The model under review builds one solid part; all positions refer to its coordinate system, in mm. Coordinates: 2 decimals unless noted, no trailing zeros. Loops run counter-clockwise (first coordinate to the right, second up) from the corner with the lowest first, then second, coordinate; pieces in that order, holes last. Notation, with made-up numbers: M 29,23 L 54,23 A32 cw 54,52 Z; hole C 27,-23 d9. An arc over 180 degrees is marked long. Use one line per item in the form item = value.
```python
from build123d import *

# Parameters (mm, degrees)
SKETCH1_R                                       = 50
BOSS_EXTRUDE1_DEPTH                             = 5
SKETCH3_R                                       = 3
CUT_EXTRUDE2_DEPTH                              = 4
CSK_FOR_M2_FLAT_HEAD_MACHINE_SCREW1_D           = 2.4
CSK_FOR_M2_FLAT_HEAD_MACHINE_SCREW1_CSINK_D     = 4.4
CSK_FOR_M2_FLAT_HEAD_MACHINE_SCREW1_CSINK_ANGLE = 90
CIRPATTERN1_COUNT                               = 6


with BuildPart() as part:
    # Sketch1 → Boss-Extrude1 (new body)
    with BuildSketch(Plane.XY):
        Circle(SKETCH1_R)
    extrude(amount=BOSS_EXTRUDE1_DEPTH)

    # Sketch3 → Cut-Extrude2 (cut)
    with BuildSketch(Plane(origin=(0, 0, 0), x_dir=(-1, 0, 0), z_dir=(0, 0, -1))):
        Circle(SKETCH3_R)
    extrude(amount=-CUT_EXTRUDE2_DEPTH, mode=Mode.SUBTRACT)

    # CSK for M2 Flat Head Machine Screw1 (through all)
    with Locations(Plane(origin=(-47.5, 0, 5), x_dir=(1, 0, 0), z_dir=(0, 0, 1))):
        with Locations((0, 0)):
            csk_for_m2_flat_head_machine_screw1 = CounterSinkHole(CSK_FOR_M2_FLAT_HEAD_MACHINE_SCREW1_D / 2, CSK_FOR_M2_FLAT_HEAD_MACHINE_SCREW1_CSINK_D / 2, counter_sink_angle=CSK_FOR_M2_FLAT_HEAD_MACHINE_SCREW1_CSINK_ANGLE)

    # CirPattern1: CSK for M2 Flat Head Machine Screw1 ×6 about axis
    cirpattern1_axis = Axis((0, 0, 0), (0, 0, 1))
    for i in range(1, CIRPATTERN1_COUNT):
        add(csk_for_m2_flat_head_machine_screw1.rotate(cirpattern1_axis, i * 360 / CIRPATTERN1_COUNT), mode=Mode.SUBTRACT)


solid = part.part
```
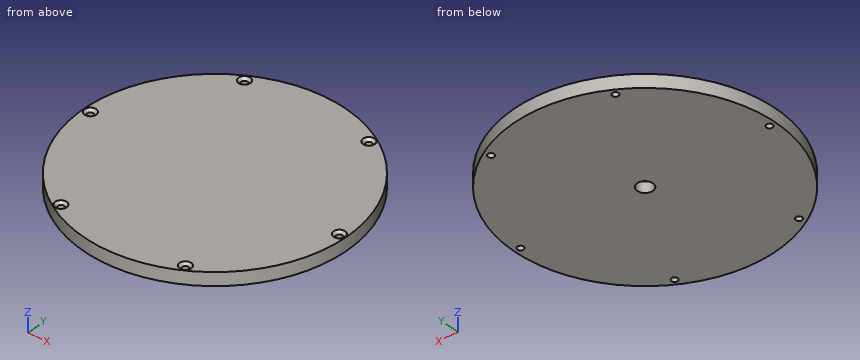
1. Add section B-B (x = -47.5). State the section outline as (y, z) points.
Response values:
outline = M -15.61,0 L -1.2,0 L -1.2,4 L -2.2,5 L -15.61,5 Z; M 1.2,0 L 15.61,0 L 15.61,5 L 2.2,5 L 1.2,4 Z
2. Wall thickness on line 1 along Y through (x, z) = (23.75, 2.35); line 2 along Y through (x, z) = (0, 3.1); line 3 along X through (y, z) = (-14, 0.6): over which ranges is each line inside the solid? List them lowest first. Write a range as from..to.
Response values:
line_1 = -44..-42.34, -39.94..39.94, 42.34..44
line_2 = -50..-3, 3..50
line_3 = -48..48
3. Insertion check: P1, Ø2, axis at y = 4.5, z = 2, coming from the -X side; P2, Ø1.4, axis at x = 47.5, y = 0, coming from the +Z side; P3, Ø5, axis at x = 0, y = 0, coming from the -Z side; P4, Ø4, axis at x = -23.75, y = -41.14, coming from the +Z side. Each pin has a flat end and moves straight along its axis. Give the tip position at first contact, or say it passes through.
Response values:
P1 = -49.88
P2 = through
P3 = 4
P4 = 4.8
4. Add section C-C (z = 2.6). State the section outline as (x, y) points, then the cut area to 3 significant figures.
Response values:
outline = C 0,0 d100; hole C -47.5,0 d2.4; hole C -23.75,-41.14 d2.4; hole C -23.75,41.14 d2.4; hole C 0,0 d6; hole C 23.75,-41.14 d2.4; hole C 23.75,41.14 d2.4; hole C 47.5,0 d2.4
area = 7,800 mm^2
5. Add section A-A (y = 0). State the section outline as (x, z) points, then the cut area to 3 significant figures.
Response values:
outline = M -50,0 L -48.7,0 L -48.7,4 L -49.7,5 L -50,5 Z; M -46.3,0 L -3,0 L -3,4 L 3,4 L 3,0 L 46.3,0 L 46.3,4 L 45.3,5 L -45.3,5 L -46.3,4 Z; M 48.7,0 L 50,0 L 50,5 L 49.7,5 L 48.7,4 Z
area = 450 mm^2
6. Add section D-D (x = 0). State the section outline as (y, z) points.
Response values:
outline = M -50,0 L -3,0 L -3,4 L 3,4 L 3,0 L 50,0 L 50,5 L -50,5 Z
